```python
from build123d import *

# Parameters (mm, degrees)
F0_R     = 5.5
F1_DEPTH = 6
F3_DEPTH = 9
F5_DEPTH = 9
F6_R     = 8
F7_DEPTH = 9


with BuildPart() as f1:
    # F0 (on Top) → F1 (new body)
    with BuildSketch(Plane.XY):
        with BuildLine():
            Line((59, 37), (0, 37))
            Line((0, 37), (0, 13))
            ThreePointArc((0, 13), (3.807612, 3.807612), (13, 0))
            Line((13, 0), (46, 0))
            ThreePointArc((46, 0), (55.192388, 3.807612), (59, 13))
            Line((59, 13), (59, 37))
        make_face()
        with Locations((13, 13)):
            Circle(F0_R, mode=Mode.SUBTRACT)
        with Locations((46, 13)):
            Circle(F0_R, mode=Mode.SUBTRACT)
    extrude(amount=F1_DEPTH)

    # F2 (on face) → F3 (join)
    with BuildSketch(Plane(origin=(0, 37, 0), x_dir=(-1, 0, 0), z_dir=(0, 1, 0))):
        Polygon((-68.103316, 53.267747), (-59, 6), (-59, 0), (0, 0), (0, 6), (-46.63881, 74.732253), align=None)
    extrude(amount=F3_DEPTH)

    # F4 (on face) → F5 (join)
    with BuildSketch(Plane(origin=(60.685531, 0, 60.685531), x_dir=(0, 1, 0), z_dir=(0.707107, 0, 0.707107))):
        with BuildLine():
            Line((46, 19.865064), (37, 19.865064))
            Line((37, 19.865064), (8, 19.865064))
            ThreePointArc((8, 19.865064), (-7.177698, 4.687367), (8, -10.490331))
            Line((8, -10.490331), (37, -10.490331))
            Line((37, -10.490331), (46, -10.490331))
            Line((46, -10.490331), (46, 19.865064))
        make_face()
    extrude(amount=F5_DEPTH)

    # F6 (on face) → F7 (cut)
    with BuildSketch(Plane(origin=(67.049492, 0, 67.049492), x_dir=(0, 1, 0), z_dir=(0.707107, 0, 0.707107))):
        with Locations((8, 4.687367)):
            Circle(F6_R)
    extrude(amount=-F7_DEPTH, mode=Mode.SUBTRACT)


solid = f1.part
```
Read the model definition and answer for the solid it produces. Units are mm, in the model's axes. A direction names the side the tool comes from. Give positions to 0.01 mm unless a question says otherwise; leave off trailing zeros. Write each loop counter-clockwise with the first axis right and the second up, starting at its lowest first coordinate (ties: lowest second). Pieces come first, ordered by that corner, then holes. Notation, with made-up numbers: (-32, 75) - (-13, 75) arc R14 cw to (-13, 101) - close; hole circle Ø4 at (-12, 14). An arc over 180 degrees is marked (long way). Write item = value, one per line. Start each with the question number.
Item 1: A tool of negligible diameter and unlimited length cuts with its end or side. For faces 1 (the flat face through (22.993, 41.437, 39.885)), 2 (the flat face through (42, 37, 33)), 3 (the flat face through (59, 29, 3)), 4 (the cylindrical face through (40.505, 13.242, 2.958)), 5 (the flat face through (29, 19, 6)), from which of +Z, -Z, +X, -X, +Y, -Y can it reach the whole face along a straight path? Write none if from no direction.
Item 2: Find section A-A (y = 25). Give the vertices of the cut face in (x, z), then the cut area to 3 significant figures.
Item 3: Find section B-B (y = 3). Give the vertices of the cut face in (x, z).
Item 4: Find the intervals of material crossed by probe 1 along Y at (x, z) = (13, 3.3); probe 2 along Y at (x, z) = (36, 35.5); probe 3 along Z at (x, y) = (44, 28), in increasing order. Write a range as [from, to].
Item 5: Find section C-C (y = 10.5). Give the vertices of the cut face in (x, z), then the cut area to 3 significant figures.
Item 6: The mould has two halves that part along Z. Classify faces 6 (the flat face through (63.6, 24.9, 70.5)), 7 (the cylindrical face through (55.091, 3.707, 2.958)), 8 (the cylindrical face through (66.12, 6.266, 61.704)): +Z half, -Z half, draft (parallel to the pull), parting line (faces both ways), or undercut.
Item 7: Each of these flat-tipped pins is pushed along its axis until it touches: P1, Ø4, axis at x = 45.5, z = 34, coming from the -Y side; P2, Ø5, axis at y = 33, z = 2, coming from the +X side; P3, Ø3, axis at x = 37, z = 2.5, coming from the -Y side. Where does it stop, or does it pass through?
Item 8: Find section D-D (z = 44.5). Give the vertices of the cut face in (x, y), then the cut area to 3 significant figures.
Response:
q1.face_1 = +Z, -X, +Y, -Y
q1.face_2 = -X, -Y
q1.face_3 = -Z, +X, +Y, -Y
q1.face_4 = -Z
q1.face_5 = +X, -X, -Y
q2.outline = (0, 0) - (59, 0) - (59, 6) - (0, 6) - close; (46.64, 74.73) - (68.1, 53.27) - (74.47, 59.63) - (53, 81.1) - close
q2.area = 627 mm²
q3.outline = (4.69, 0) - (54.31, 0) - (54.31, 6) - (4.69, 6) - close; (47.24, 74.13) - (52.96, 68.42) - (59.32, 74.78) - (53.6, 80.5) - close; (61.79, 59.58) - (67.5, 53.87) - (73.87, 60.23) - (68.15, 65.95) - close
q4.probe_1 = [0, 7.5], [18.5, 46]
q4.probe_2 = [37, 46]
q4.probe_3 = [0, 6]
q5.outline = (0.24, 0) - (8.1, 0) - (8.1, 6) - (0.24, 6) - close; (17.9, 0) - (41.1, 0) - (41.1, 6) - (17.9, 6) - close; (46.64, 74.73) - (52, 69.37) - (58.36, 75.74) - (53, 81.1) - close; (50.9, 0) - (58.76, 0) - (58.76, 6) - (50.9, 6) - close; (62.74, 58.63) - (68.1, 53.27) - (74.47, 59.63) - (69.11, 64.99) - close
q5.area = 370 mm²
q6.face_6 = +Z half
q6.face_7 = draft
q6.face_8 = undercut
q7.P1 = 37
q7.P2 = 59
q7.P3 = 0
q8.outline = (26.12, 37) - (66.41, 37) - (66.41, 46) - (26.12, 46) - close
q8.area = 363 mm²
